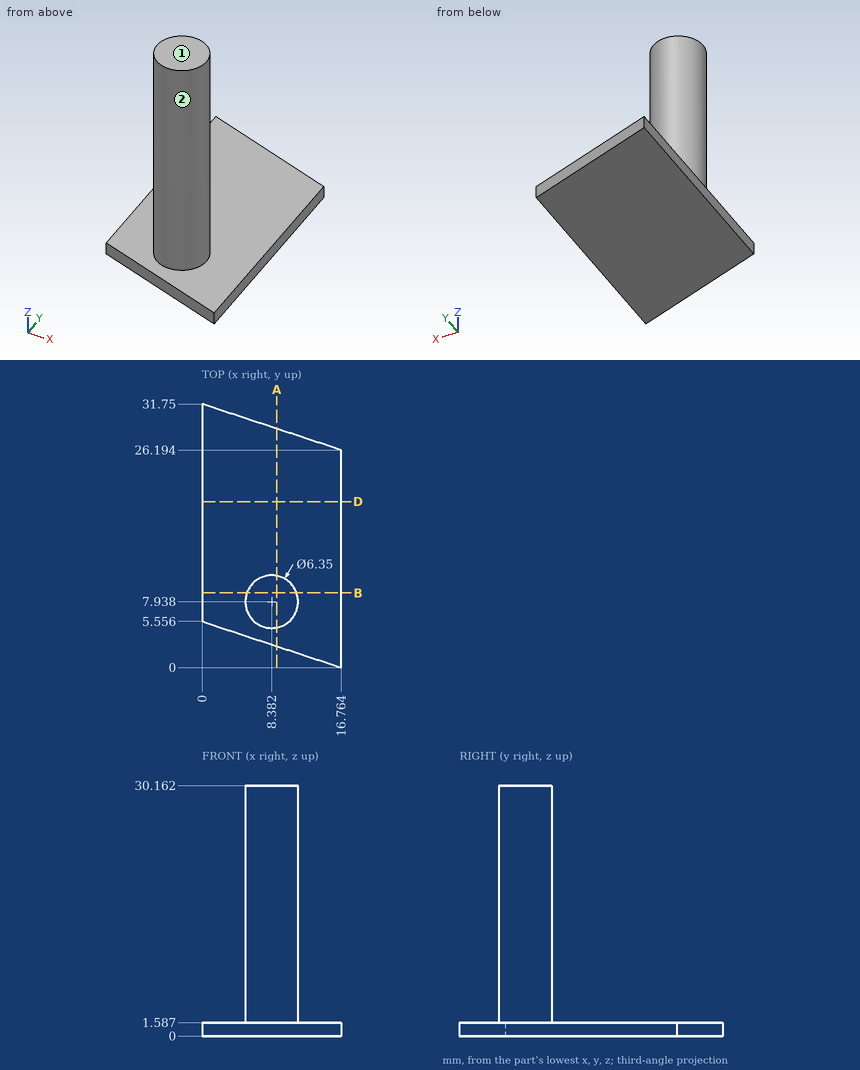
The figure shows three views and two pictorial views of one solid part (mm, origin at its lowest corner). Answer the questions. A direction names the side the tool comes from. Round coordinates to 2 decimals unless told otherwise and drop trailing zeros. Loops run counter-clockwise (first coordinate to the right, second up) from the corner with the lowest first, then second, coordinate; pieces in that order, holes last. Notation, with made-up numbers: M 13.5,-32 L 50.5,-32 A5 cw 50.5,-27 Z; hole C 23,-26.5 d9. An arc over 180 degrees is marked long. Return JSON: item names as keys, results as strings.
Q1. Find section B-B, the plane y = 9. Determine the outline of the cut face in (x, z) (1 decimal), plus the area to 3 significant figures.
Results list:
{"outline": "M 0,0 L 16.8,0 L 16.8,1.6 L 11.4,1.6 L 11.4,30.2 L 5.4,30.2 L 5.4,1.6 L 0,1.6 Z", "area": "198 mm2"}
Q2. Which of the six approach directions +Z, -Z, +X, -X, +Y, -Y give full straight-line access (tool end or side, diameter ignored) to the marked faces 1 and 2?
Results list:
{"face 1": "+Z, +X, -X, +Y, -Y", "face 2": "+Z"}
Q3. Find section A-A, the plane x = 9. Determine the outline of the cut face in (y, z).
Results list:
{"outline": "M 2.57,0 L 28.77,0 L 28.77,1.59 L 11.05,1.59 L 11.05,30.16 L 4.82,30.16 L 4.82,1.59 L 2.57,1.59 Z"}
Q4. Each of these flat-tipped pins is pushed along its axis until it touches: pin 1 Ø12 at (y, z) = (6.5, 20.5) entering from -X; pin 2 Ø5 at (x, z) = (10, 19) entering from +Y; pin 3 Ø8.5 at (x, y) = (7.5, 23.5) entering from +Z. Where does it stop, or does it pass through?
Results list:
{"pin 1": "stops at x = 5.21", "pin 2": "stops at y = 11.11", "pin 3": "stops at z = 1.59"}
Q5. Find section D-D, the plane y = 20. Determine the outline of the cut face in (x, z) (1 decimal).
Results list:
{"outline": "M 0,0 L 16.8,0 L 16.8,1.6 L 0,1.6 Z"}
Q6. Find the intervals of material crossed by line 1 along Z through (x, y) = (6, 11); line 2 along Y through (x, z) = (8.25, 11.5) (1 decimal); line 3 along X through (y, z) = (6.5, 20.5), in increasing order. Write a range as from..to.
Results list:
{"line 1": "z = 0..1.59", "line 2": "y = 4.8..11.1", "line 3": "x = 5.55..11.21"}
